Could you check a few things on this model? Use its own coordinates, in mm. A direction names the side the tool comes from. Coordinates: 2 decimals unless noted, no trailing zeros. Write each loop counter-clockwise with the first axis right and the second up, starting at its lowest first coordinate (ties: lowest second). Pieces come first, ordered by that corner, then holes. Notation, with made-up numbers: M -19.5,33 L -6.5,33 A11 cw -6.5,38 Z; hole C 51.25,65.5 d4. An arc over 180 degrees is marked long. Answer as CSV lines item,"result". Start each with the question number.
Item 1: On a 3-axis mill with a long thin cutter (end or side, diameter ignored), from which of +Z, -Z, +X, -X, +Y, -Y can I reach the whole of each face in a straight line? I mean faces 1 (the flat face through (26.8, 15, 11)), 2 (the flat face through (20.7, 3.5, -10.5)), 3 (the flat face through (23.8, 15, -1)). Say none if no direction works.
Item 2: Suppose I cut it at C-C, the plane z = 7.25. Write out the boundary of the cut face in (x, y) (3 decimals), and give its area (3 significant figures).
Item 3: If I drill on line 1 along Z through (x, y) = (17.2, 26.5); line 2 along Y through (x, z) = (20, 11.5); line 3 along Y through (x, z) = (17.75, 12), over which ranges is the centre line in solid material (lowest first)? Write a range as [from, to].
Item 4: Suppose I cut it at B-B, the plane x = 16.6. State how many separate pieces and enclosed holes the cut face has, and give its area (3 significant figures).
Item 5: I'm going to push flat-ended pins straight in: P1, Ø2.5, axis at y = 26.5, z = 10.5, coming from the -X side; P2, Ø12, axis at y = 6, z = 3, coming from the -X side; P3, Ø5, axis at x = 25.5, z = -1, coming from the -Y side. Where does each tip first touch, or does it pass through?
```python
from build123d import *

# Parameters (mm, degrees)
SKETCH_1_R                 = 2.9
EXTRUDE_1_DEPTH            = 30
SKETCH_2_W                 = 27.5
SKETCH_2_H                 = 30
EXTRUDE_2_DEPTH            = 17
CUT_EXTRUDE_1_REACH        = 39.833
SKETCH_3_W                 = 27.5
SKETCH_3_H                 = 19.8
SKETCH_4_W                 = 27.5
SKETCH_4_H                 = 30
SKETCH_4_W_2               = 23
SKETCH_4_H_2               = 27.5
CUT_EXTRUDE_2_DEPTH        = 4.5
CHAMFER_1_SIZE             = 3
SKETCH_5_W                 = 20.5
SKETCH_5_H                 = 13
CUT_EXTRUDE_3_DEPTH        = 3
SKETCH_6_R                 = 7.5
SKETCH_6_R_2               = 2.9
EXTRUDE_3_DEPTH            = 2.2
CHAMFER_2_SIZE             = 2
CHAMFER_2_OF_MIRROR_1_SIZE = 2
CUT_EXTRUDE_4_REACH        = 52.113
SKETCH_7_W                 = 25
SKETCH_7_H                 = 34.4
SKETCH_8_W                 = 25.25
SKETCH_8_H                 = 27.75
SKETCH_8_W_2               = 24.85
SKETCH_8_H_2               = 27.35
EXTRUDE_4_DEPTH            = 0.5
SKETCH_9_W                 = 24.85
SKETCH_9_H                 = 27.35
CUT_EXTRUDE_5_DEPTH        = 5
SKETCH_10_R                = 4.5
EXTRUDE_5_DEPTH            = 5
SKETCH_11_R                = 2.85
SKETCH_11_R_2              = 0.85
EXTRUDE_6_DEPTH            = 5


with BuildPart() as part:
    # 草图1 → 凸台-拉伸1 (new body)
    with BuildSketch(Plane(origin=(0, 0, 0), x_dir=(1, 0, 0), z_dir=(0, 1, 0))):
        with BuildLine():
            Line((-0.305751289, 8.694625705), (9.8, 9.05))
            Line((9.8, 9.05), (9.8, -9.05))
            Line((9.8, -9.05), (-0.305751289, -8.694625705))
            ThreePointArc((-0.305751289, -8.694625705), (-8.7, 0), (-0.305751289, 8.694625705))
        make_face()
        with Locations(Location((0, 0, 0), (0, 0, 270))):
            Circle(SKETCH_1_R, mode=Mode.SUBTRACT)
    extrude(amount=EXTRUDE_1_DEPTH)

    # 草图2 → 凸台-拉伸2 (add)
    with BuildSketch(Plane(origin=(9.8, 0, 0), x_dir=(0, 0, -1), z_dir=(1, 0, 0))):
        with Locations((0, 15)):
            Rectangle(SKETCH_2_W, SKETCH_2_H)
    extrude(amount=EXTRUDE_2_DEPTH)

    # 草图3 → 切除-拉伸1 (cut, up to next)
    with BuildSketch(Plane.ZY.offset(-9.8), mode=Mode.PRIVATE) as cut_extrude_1_sk1:
        with Locations((0, 15)):
            Rectangle(SKETCH_3_W, SKETCH_3_H)
    cut_extrude_1_tool1 = extrude(cut_extrude_1_sk1.sketch, amount=CUT_EXTRUDE_1_REACH, mode=Mode.PRIVATE) & part.part
    add(cut_extrude_1_tool1.solids().sort_by_distance((9.8, 15, 0))[0], mode=Mode.SUBTRACT)

    # 草图4 → 切除-拉伸2 (cut)
    with BuildSketch(Plane(origin=(26.8, 0, 0), x_dir=(0, 0, -1), z_dir=(1, 0, 0))):
        with Locations((0, 15)):
            Rectangle(SKETCH_4_W, SKETCH_4_H)
        with Locations((0, 15)):
            Rectangle(SKETCH_4_W_2, SKETCH_4_H_2, mode=Mode.SUBTRACT)
    extrude(amount=-CUT_EXTRUDE_2_DEPTH, mode=Mode.SUBTRACT)

    # 倒角1
    chamfer_1_edges = [part.edges().sort_by_distance(p)[0] for p in [
        (26.8, 15, -11.5),
    ]]
    chamfer(chamfer_1_edges, length=CHAMFER_1_SIZE)

    # 草图5 → 切除-拉伸3 (cut)
    with BuildSketch(Plane(origin=(26.8, 0, 0), x_dir=(0, 0, -1), z_dir=(1, 0, 0))):
        with Locations((1.25, 15)):
            Rectangle(SKETCH_5_W, SKETCH_5_H)
    extrude(amount=-CUT_EXTRUDE_3_DEPTH, mode=Mode.SUBTRACT)

    # 草图6 → 凸台-拉伸3 (add)
    with BuildSketch(Plane(origin=(0, 30, 0), x_dir=(1, 0, 0), z_dir=(0, 1, 0))):
        with Locations(Location((0, 0, 0), (0, 0, 270))):
            Circle(SKETCH_6_R)
        with Locations(Location((0, 0, 0), (0, 0, 270))):
            Circle(SKETCH_6_R_2, mode=Mode.SUBTRACT)
    extrude_3 = extrude(amount=EXTRUDE_3_DEPTH)

    # 倒角2
    chamfer_2_edges = [part.edges().sort_by_distance(p)[0] for p in [
        (0, 32.2, -7.5),
    ]]
    chamfer(chamfer_2_edges, length=CHAMFER_2_SIZE)

    # 镜向1: 凸台-拉伸3 across plane
    add(extrude_3.mirror(Plane(origin=(0, 15, 0), x_dir=(0, 0, 1), z_dir=(0, -1, 0))))

    # 倒角2 of 镜向1
    chamfer_2_of_mirror_1_edges = [part.edges().sort_by_distance(p)[0] for p in [
        (0, -2.2, -7.5),
    ]]
    chamfer(chamfer_2_of_mirror_1_edges, length=CHAMFER_2_OF_MIRROR_1_SIZE)

    # 草图7 → 切除-拉伸4 (cut, up to next)
    with BuildSketch(Plane(origin=(0, 0, -13.75), x_dir=(-1, 0, 0), z_dir=(0, 0, -1)), mode=Mode.PRIVATE) as cut_extrude_4_sk1:
        with Locations((-3.2, 15)):
            Rectangle(SKETCH_7_W, SKETCH_7_H)
    cut_extrude_4_tool1 = extrude(cut_extrude_4_sk1.sketch, amount=-CUT_EXTRUDE_4_REACH, mode=Mode.PRIVATE) & part.part
    add(cut_extrude_4_tool1.solids().sort_by_distance((3.2, 15, -13.75))[0], mode=Mode.SUBTRACT)

    # 草图8 → 凸台-拉伸4 (add)
    with BuildSketch(Plane.ZY.offset(-15.7)):
        with Locations((0, 15)):
            Rectangle(SKETCH_8_W, SKETCH_8_H)
        with Locations((0, 15)):
            Rectangle(SKETCH_8_W_2, SKETCH_8_H_2, mode=Mode.SUBTRACT)
    extrude(amount=EXTRUDE_4_DEPTH)

    # 草图9 → 切除-拉伸5 (cut)
    with BuildSketch(Plane.ZY.offset(-15.7)):
        with Locations((0, 15)):
            Rectangle(SKETCH_9_W, SKETCH_9_H)
    extrude(amount=-CUT_EXTRUDE_5_DEPTH, mode=Mode.SUBTRACT)

    # 草图10 → 凸台-拉伸5 (add)
    with BuildSketch(Plane.XY.offset(13.75)):
        with Locations((16.6, 15)):
            Circle(SKETCH_10_R)
    extrude(amount=-EXTRUDE_5_DEPTH)

    # 草图11 → 凸台-拉伸6 (add)
    # profile 1 of 4: a face of its own
    with BuildSketch(Plane.ZY.offset(-15.7)):
        with Locations((-10.5, 26.5)):
            Circle(SKETCH_11_R)
        with Locations(Location((-10.5, 26.5, 0), (0, 0, 270))):
            Circle(SKETCH_11_R_2, mode=Mode.SUBTRACT)
    # profile 2 of 4: a face of its own
    with BuildSketch(Plane.ZY.offset(-15.7)):
        with Locations((10.5, 26.5)):
            Circle(SKETCH_11_R)
        with Locations(Location((10.5, 26.5, 0), (0, 0, 270))):
            Circle(SKETCH_11_R_2, mode=Mode.SUBTRACT)
    # profile 3 of 4: a face of its own
    with BuildSketch(Plane.ZY.offset(-15.7)):
        with Locations((-10.5, 3.5)):
            Circle(SKETCH_11_R)
        with Locations(Location((-10.5, 3.5, 0), (0, 0, 270))):
            Circle(SKETCH_11_R_2, mode=Mode.SUBTRACT)
    # profile 4 of 4: a face of its own
    with BuildSketch(Plane.ZY.offset(-15.7)):
        with Locations((10.5, 3.5)):
            Circle(SKETCH_11_R)
        with Locations(Location((10.5, 3.5, 0), (0, 0, 270))):
            Circle(SKETCH_11_R_2, mode=Mode.SUBTRACT)
    extrude(amount=-EXTRUDE_6_DEPTH)


solid = part.part
```
Ans:
1,face 1,"+Z, -Z, +X, +Y, -Y"
1,face 2,"-X"
1,face 3,"-Z, +X"
2,outline,"M 15.2,1.125 L 15.7,1.125 L 15.7,0 L 22.3,0 L 22.3,1.25 L 26.8,1.25 L 26.8,8.5 L 23.8,8.5 L 23.8,21.5 L 26.8,21.5 L 26.8,28.75 L 22.3,28.75 L 22.3,30 L 15.7,30 L 15.7,28.875 L 15.2,28.875 L 15.2,28.675 L 20.7,28.675 L 20.7,1.325 L 15.2,1.325 Z"
2,area,"146 mm^2"
3,line 1,"z = [-13.75, -11.35], [-9.65, -7.65], [7.65, 9.65], [11.35, 13.75]"
3,line 2,"y = [0, 6.17], [12.05, 17.95], [23.83, 30]"
3,line 3,"y = [0, 5.92], [10.65, 19.35], [24.08, 30]"
4,separate pieces,"1"
4,enclosed holes,"9"
4,area,"254 mm^2"
5,P1,"stops at x = 15.7"
5,P2,"stops at x = 15.2"
5,P3,"stops at y = 1.25"
